CAD build for the part. Positions are in the model's coordinates, mm. A direction names the side the tool comes from. Round coordinates to 2 decimals unless told otherwise and drop trailing zeros. Answer in a Markdown table with one row per item.
```python
from build123d import *

# Parameters (mm, degrees)
SKETCH1_W             = 50
SKETCH1_H             = 180
SKETCH1_R             = 2.75
SKETCH1_R_2           = 2
BOSS_EXTRUDE1_DEPTH   = 10
SKETCH2_R             = 5
CUT_EXTRUDE1_DEPTH    = 5
M4_TAPPED_HOLE1_D     = 3.3
M4_TAPPED_HOLE2_D     = 3.3
M4_TAPPED_HOLE2_DEPTH = 8
M4_TAPPED_HOLE2_TIP   = 0.991420021


with BuildPart() as part:
    # Sketch1 → Boss-Extrude1 (new body)
    with BuildSketch(Plane.XY):
        with Locations((-10.981308411, -54.193925234)):
            Rectangle(SKETCH1_W, SKETCH1_H)
        with Locations((-10.981308411, -119.193925234)):
            Circle(SKETCH1_R, mode=Mode.SUBTRACT)
        with Locations((-10.981308411, -64.193925234)):
            Circle(SKETCH1_R, mode=Mode.SUBTRACT)
        with Locations((-10.981308411, -9.193925234)):
            Circle(SKETCH1_R, mode=Mode.SUBTRACT)
        with Locations((9.018691589, 20.806074766)):
            Circle(SKETCH1_R_2, mode=Mode.SUBTRACT)
        with Locations((9.018691589, -19.193925234)):
            Circle(SKETCH1_R_2, mode=Mode.SUBTRACT)
    extrude(amount=BOSS_EXTRUDE1_DEPTH)

    # Sketch2 → Cut-Extrude1 (cut)
    with BuildSketch(Plane.XY.offset(10)):
        with Locations((-10.981308411, -9.193925234)):
            Circle(SKETCH2_R)
        with Locations((-10.981308411, -64.193925234)):
            Circle(SKETCH2_R)
        with Locations((-10.981308411, -119.193925234)):
            Circle(SKETCH2_R)
    extrude(amount=-CUT_EXTRUDE1_DEPTH, mode=Mode.SUBTRACT)

    # M4 Tapped Hole1 (through all)
    with Locations(Plane.XY.offset(10)):
        with Locations((-0.981308411, -19.193925234), (-20.981308411, -19.193925234), (-20.981308411, 20.806074766), (-0.981308411, 20.806074766)):
            Hole(M4_TAPPED_HOLE1_D / 2)

    # M4 Tapped Hole2
    with Locations(Plane(origin=(0, -144.193925234, 0), x_dir=(-1, 0, 0), z_dir=(0, -1, 0))):
        with Locations((29.981308411, -5), (-8.018691589, -5)):
            Hole(M4_TAPPED_HOLE2_D / 2, depth=M4_TAPPED_HOLE2_DEPTH)
            with Locations((0, 0, -(M4_TAPPED_HOLE2_DEPTH + M4_TAPPED_HOLE2_TIP / 2))):  # 118° drill point
                Cone(0, M4_TAPPED_HOLE2_D / 2, M4_TAPPED_HOLE2_TIP, mode=Mode.SUBTRACT)


solid = part.part
```
Q1. 3-axis set-ups, long thin cutter, end or side, ignore diameter. For faces 4 (the cylindrical face through (-22.505, 20.174, 4.93)), 5 (the cylindrical face through (9.543, -140.138, 5.632)), 6 (the cylindrical face through (-12.065, -124.075, 7.535)): which of +Z, -Z, +X, -X, +Y, -Y reach the whole face in a straight line?
Computed:
| item | result |
|---|---|
| face 4 | +Z, -Z |
| face 5 | -Y |
| face 6 | +Z |
Q2. Drill centre lines: line 1 (Y direction, x = 8, z = 3); line 2 (Y direction, x = 10.5, z = 8); line 3 (Y direction, x = -13, z = 2). Where is each one in solid material? Low to high.
Computed:
| item | result |
|---|---|
| line 1 | y = -144.19 to -20.92, -17.47 to 19.08, 22.53 to 35.81 |
| line 2 | y = -144.19 to -20.54, -17.85 to 19.46, 22.15 to 35.81 |
| line 3 | y = -144.19 to -121.06, -117.33 to -66.06, -62.33 to -11.06, -7.33 to 35.81 |
Q3. Flat gauge pin, fed straight in: pin 1 (3 mm diameter, centred on x = -10, y = -63, fed in from +Z). Where does the tip first touch, or does it go through?
Computed:
| item | result |
|---|---|
| pin 1 | stops at z = 5 |
Q4. Pull direction Y, two halves, no side cores. Call faces 1 (the flat face through (14.019, -55, 5)), 2 (the conical face through (-29.7, -135.37, 4.99)), 3 (the cylindrical face through (-11.339, -6.467, 2.465)): released by +Y, released by -Y, zero draft, split by the parting line, or undercut.
Computed:
| item | result |
|---|---|
| face 1 | zero draft |
| face 2 | released by -Y |
| face 3 | undercut |
